Verification items for the finished model (mm, model axes). Give positions to 0.01 mm unless a question says otherwise; leave off trailing zeros. Order: outer loops, then holes, each group sorted by start corner. A loop starts at its lowest first (then second) coordinate and runs counter-clockwise, first axis right, second up.
(1) Sectioned sample at A-A on x = 0. Record the cut outline in (y, z) (1 decimal).
(2) Gauge pin test, flat ends, axial feed: pin 1 (2 mm diameter, centred on x = -1.5, y = 7.5, fed in from +Z); pin 2 (2 mm diameter, centred on x = 0.5, z = 2.5, fed in from +Y); pin 3 (4 mm diameter, centred on y = 6.5, z = 2.5, fed in from +X); pin 4 (1.5 mm diameter, centred on x = 2, y = 7.5, fed in from +Z). Record the tip position at first contact, or that the pin passes through.
(3) Sectioned sample at B-B on y = 5.25. Record the cut outline in (x, z), plus the area to 3 significant figures.
(4) Sectioned sample at D-D on y = 7. Record the cut outline in (x, z).
(5) Scan lines: L1, parallel to Y at x = 3.75, z = 0; L2, parallel to Y at x = -2.25, z = 1.25; L3, parallel to X at y = 4.5, z = -1.5. Record each from-to range of solid material in increasing order.
(6) Sectioned sample at C-C on z = 0. Record the cut outline in (x, y), plus the area to 3 significant figures.
```python
from build123d import *

# Parameters (mm, degrees)
F0_R          = 3.96875
F1_DEPTH      = 11.0998
F3_DEPTH      = 25.4
F3_DEPTH_BACK = 25.4
F4_SIZE2      = 1.5875
F4_SIZE       = 1.5875
F7_DEPTH      = 25.4
F7_DEPTH_BACK = 25.4


with BuildPart() as f1:
    # F0 (on Front) → F1 (new body)
    with BuildSketch(Plane.XZ):
        Circle(F0_R)
    extrude(amount=-F1_DEPTH)

    # F2 (on Right) → F3 (cut, two sides)
    with BuildSketch(Plane.YZ) as f3_sk:
        Polygon((11.0998, -21.43125), (11.0998, 3.96875), (-3.5648968374, -21.43125), align=None)
    extrude(amount=-F3_DEPTH, mode=Mode.SUBTRACT)
    extrude(f3_sk.sketch, amount=F3_DEPTH_BACK, mode=Mode.SUBTRACT)

    # F4
    f4_edges = [f1.edges().sort_by_distance(p)[0] for p in [
        (-3.96875, 0, 0),
    ]]
    chamfer(f4_edges, length=F4_SIZE, length2=F4_SIZE2)

    # F6 (on offset) → F7 (cut, two sides)
    with BuildSketch(Plane.YZ) as f7_sk:
        with BuildLine():
            ThreePointArc((8.350169343, 3.96875), (9.7249846715, 3.175), (9.7249846715, 1.5875))
            Line((9.7249846715, 1.5875), (11.0998, 3.96875))
            Line((11.0998, 3.96875), (8.350169343, 3.96875))
        make_face()
    extrude(amount=-F7_DEPTH, mode=Mode.SUBTRACT)
    extrude(f7_sk.sketch, amount=F7_DEPTH_BACK, mode=Mode.SUBTRACT)


solid = f1.part
```
Ans:
1. outline: (0, -2.4) - (1.6, -4) - (6.5, -4) - (9.7, 1.6) arc R1.6 ccw to (8.4, 4) - (1.6, 4) - (0, 2.4) - close
2. pin 1: stops at z = 3.94
2. pin 2: stops at y = 9.94
2. pin 3: stops at x = 3.94
2. pin 4: stops at z = 3.77
3. outline: circle Ø7.94 at (0, 0)
3. area: 49.5 mm2
4. outline: (-2.44, -3.13) - (2.44, -3.13) arc R3.97 ccw (long way) to start
5. L1: y = 1.37 to 8.81
5. L2: y = 0.19 to 9.53
5. L3: x = -3.67 to 3.67
6. outline: (-3.97, 1.59) - (-2.38, 0) - (2.38, 0) - (3.97, 1.59) - (3.97, 8.81) - (-3.97, 8.81) - close
6. area: 67.4 mm2
